```python
from build123d import *

# Parameters (mm, degrees)
F2_SIZE  = 0.3
F4_DEPTH = 2


with BuildPart() as f1:
    # F0 (on Top) → F1 (revolve)
    with BuildSketch(Plane.XY):
        Polygon((0, 3.5), (0, 0), (16, 0), (16, 2), (4, 2), (4, 3.5), align=None)
    revolve(axis=Axis((8, 0, 0), (-1, 0, 0)))

    # F2
    f2_edges = [f1.edges().sort_by_distance(p)[0] for p in [
        (0, -3.5, 0),
        (16, -2, 0),
    ]]
    chamfer(f2_edges, length=F2_SIZE)

    # F3 (on face) → F4 (cut)
    with BuildSketch(Plane(origin=(0, 0, 0), x_dir=(0, -1, 0), z_dir=(-1, 0, 0))):
        Polygon((1.525, 0.880459), (0, 1.760918), (-1.525, 0.880459), (-1.525, -0.880459), (0, -1.760918), (1.525, -0.880459), align=None)
    extrude(amount=-F4_DEPTH, mode=Mode.SUBTRACT)


solid = f1.part
```
Design review of the part built by this model. Coordinates are the model's own, in mm. A direction names the side the tool comes from. Give positions to 0.01 mm unless a question says otherwise; leave off trailing zeros. Loops run counter-clockwise (first coordinate to the right, second up) from the corner with the lowest first, then second, coordinate; pieces in that order, holes last. Notation, with made-up numbers: (-25.75, 54.5) -> (17.25, 54.5) arc R29 ccw to (17.25, 81.5) -> close; hole circle Ø3 at (-29.5, -38). An arc over 180 degrees is marked (long way). One line per item, written item: value.
Q1. We need section B-B on x = 9.25. Give the boundary of the cut face in (y, z), and give its area (3 significant figures).
Numbers:
outline: circle Ø4 at (0, 0)
area: 12.6 mm^2
Q2. We need section A-A on z = 0. Give the boundary of the cut face in (x, y) (3 decimals), and give its area (3 significant figures).
Numbers:
outline: (0, -3.2) -> (0.3, -3.5) -> (4, -3.5) -> (4, -2) -> (15.7, -2) -> (16, -1.7) -> (16, 1.7) -> (15.7, 2) -> (4, 2) -> (4, 3.5) -> (0.3, 3.5) -> (0, 3.2) -> (0, 1.525) -> (2, 1.525) -> (2, -1.525) -> (0, -1.525) -> close
area: 69.7 mm^2
Q3. Draft analysis for pull direction Y (two halves, no side actions). For faces 4 (the flat face through (2, 0, 0)), 5 (the flat face through (1, 0.8, 1.3)), 6 (the cylindrical face through (2.124, 3.233, 1.341)), 7 (the flat face through (0, -0.8, -1.5)), state which applies: pulls with the +Y half, pulls with the -Y half, needs draft (parallel to the pull), parting line crosses it, or undercut.
Numbers:
face 4: undercut
face 5: undercut
face 6: parting line crosses it
face 7: needs draft
Q4. For pin 1 Ø1 at (x, z) = (12.5, 2) entering from +Y; pin 2 Ø4 at (x, z) = (10.5, 0.5) entering from +Y; pin 3 Ø2 at (x, z) = (7.5, -1.5) entering from +Y, all flat-tipped, find the tip position at first contact; note any pin that passes through.
Numbers:
pin 1: stops at y = 1.32
pin 2: stops at y = 2
pin 3: stops at y = 1.94
Q5. Machinability: for faces 1 (the flat face through (16, 0, 0)), 2 (the cylindrical face through (10, 0, 2)), 3 (the flat face through (1, -1.525, 0)), which of the approach directions +Z, -Z, +X, -X, +Y, -Y give a long, thin tool a straight path to every point of the face, cutting with its end or side? Answer none if there is none.
Numbers:
face 1: +Z, -Z, +X, +Y, -Y
face 2: +X
face 3: -X
Q6. For L1, parallel to X at y = -2.25, z = -2; L2, parallel to X at y = 0.75, z = 1; L3, parallel to Z at x = 2.75, y = -1.75, list the stretches that pass through material, from the lowest coordinate up.
Numbers:
L1: x = 0 to 4
L2: x = 2 to 16
L3: z = -3.03 to 3.03
